```python
from build123d import *

# Parameters (mm, degrees)
AUFSATZ_LINEAR_AUSTRAGEN1_DEPTH      = 7.5
AUFSATZ_LINEAR_AUSTRAGEN1_DEPTH_BACK = 11
SKIZZE1_R                            = 12.5
SKIZZE1_R_2                          = 1.55
SCHNITT_LINEAR_AUSTRAGEN1_DEPTH      = 4.5
AUFSATZ_LINEAR_AUSTRAGEN2_DEPTH      = 5
SCHNITT_LINEAR_AUSTRAGEN4_DEPTH      = 22.650635095
SCHNITT_LINEAR_AUSTRAGEN4_DEPTH_BACK = 22.650635095
SCHNITT_LINEAR_AUSTRAGEN5_DEPTH      = 10
SCHNITT_LINEAR_AUSTRAGEN5_DEPTH_BACK = 22.650635095
SKIZZE5_OUTSIDE_W                    = 35.49
SKIZZE5_OUTSIDE_H                    = 35.49
SKIZZE5_OUTSIDE_W_2                  = 20
SKIZZE5_OUTSIDE_H_2                  = 30
VERRUNDUNG1_R                        = 1.2
VERRUNDUNG2_R                        = 1


with BuildPart() as part:
    # Skizze1 → Aufsatz-Linear austragen1 (new, two sides: drawn at the far end of the back side and taken through both)
    with BuildSketch(Plane.XY.offset(-AUFSATZ_LINEAR_AUSTRAGEN1_DEPTH_BACK)):
        Circle(SKIZZE1_R)
        with Locations((0, 8)):
            Circle(SKIZZE1_R_2, mode=Mode.SUBTRACT)
        with Locations(Location((0, -8, 0), (0, 0, 180))):
            Circle(SKIZZE1_R_2, mode=Mode.SUBTRACT)
    extrude(amount=AUFSATZ_LINEAR_AUSTRAGEN1_DEPTH + AUFSATZ_LINEAR_AUSTRAGEN1_DEPTH_BACK)

    # Skizze2 → Schnitt-Linear austragen1 (cut)
    with BuildSketch(Plane(origin=(0, 0, -11), x_dir=(-1, 0, 0), z_dir=(0, 0, -1))):
        with BuildLine():
            Line((-9, -4), (-9, 4))
            ThreePointArc((-9, 4), (-8.707106781, 4.707106781), (-8, 5))
            Line((-8, 5), (8, 5))
            ThreePointArc((8, 5), (8.707106781, 4.707106781), (9, 4))
            Line((9, 4), (9, -4))
            ThreePointArc((9, -4), (8.707106781, -4.707106781), (8, -5))
            Line((8, -5), (-8, -5))
            ThreePointArc((-8, -5), (-8.707106781, -4.707106781), (-9, -4))
        make_face()
    extrude(amount=-SCHNITT_LINEAR_AUSTRAGEN1_DEPTH, mode=Mode.SUBTRACT)

    # Skizze3 → Aufsatz-Linear austragen2 (add)
    with BuildSketch(Plane.XY.offset(7.5)):
        with BuildLine():
            Line((-8, 5), (8, 5))
            ThreePointArc((8, 5), (8.707106781, 4.707106781), (9, 4))
            Line((9, 4), (9, -4))
            ThreePointArc((9, -4), (8.707106781, -4.707106781), (8, -5))
            Line((8, -5), (-8, -5))
            ThreePointArc((-8, -5), (-8.707106781, -4.707106781), (-9, -4))
            Line((-9, -4), (-9, 4))
            ThreePointArc((-9, 4), (-8.707106781, 4.707106781), (-8, 5))
        make_face()
    extrude(amount=AUFSATZ_LINEAR_AUSTRAGEN2_DEPTH)

    # Skizze4 → Schnitt-Linear austragen4 (cut, two sides: drawn at the far end of the back side and taken through both)
    with BuildSketch(Plane.XY.offset(-SCHNITT_LINEAR_AUSTRAGEN4_DEPTH_BACK)):
        with BuildLine():
            Line((-6.5, -3), (6.5, -3))
            ThreePointArc((6.5, -3), (7.207106781, -2.707106781), (7.5, -2))
            Line((7.5, -2), (7.5, 2))
            ThreePointArc((7.5, 2), (7.207106781, 2.707106781), (6.5, 3))
            Line((6.5, 3), (-6.5, 3))
            ThreePointArc((-6.5, 3), (-7.207106781, 2.707106781), (-7.5, 2))
            Line((-7.5, 2), (-7.5, -2))
            ThreePointArc((-7.5, -2), (-7.207106781, -2.707106781), (-6.5, -3))
        make_face()
    extrude(amount=SCHNITT_LINEAR_AUSTRAGEN4_DEPTH + SCHNITT_LINEAR_AUSTRAGEN4_DEPTH_BACK, mode=Mode.SUBTRACT)

    # Skizze5 outside → Schnitt-Linear austragen5 (cut, two sides: drawn at the far end of the back side and taken through both)
    with BuildSketch(Plane.XY.offset(-SCHNITT_LINEAR_AUSTRAGEN5_DEPTH_BACK)):
        Rectangle(SKIZZE5_OUTSIDE_W, SKIZZE5_OUTSIDE_H)
        Rectangle(SKIZZE5_OUTSIDE_W_2, SKIZZE5_OUTSIDE_H_2, mode=Mode.SUBTRACT)
    extrude(amount=SCHNITT_LINEAR_AUSTRAGEN5_DEPTH + SCHNITT_LINEAR_AUSTRAGEN5_DEPTH_BACK, mode=Mode.SUBTRACT)

    # Verrundung1
    verrundung1_edges = [part.edges().sort_by_distance(p)[0] for p in [
        (-8.707106781, 4.707106781, -11),
        (-8.707106781, -4.707106781, -11),
        (0, -5, -11),
        (8.707106781, -4.707106781, -11),
        (8.707106781, 4.707106781, -11),
        (0, 5, -11),
    ]]
    fillet(verrundung1_edges, radius=VERRUNDUNG1_R)

    # Verrundung2
    verrundung2_edges = [part.edges().sort_by_distance(p)[0] for p in [
        (8.707106781, 4.707106781, 7.5),
        (0, 5, 7.5),
        (-8.707106781, 4.707106781, 7.5),
        (-9, 0, 7.5),
        (-8.707106781, -4.707106781, 7.5),
        (0, -5, 7.5),
        (8.707106781, -4.707106781, 7.5),
        (9, 0, 7.5),
    ]]
    fillet(verrundung2_edges, radius=VERRUNDUNG2_R - 0.0001)  # a hair under: the kernel refuses the full size


solid = part.part
```
The listing builds one solid part. Answer for the finished solid, in the listing's coordinates (mm). A direction names the side the tool comes from. Coordinates: 2 decimals unless noted, no trailing zeros. Write each loop counter-clockwise with the first axis right and the second up, starting at its lowest first coordinate (ties: lowest second). Pieces come first, ordered by that corner, then holes.
Q1. Section A-A, the plane x = 0 is taken. Write down the section's boundary in (y, z), then the cut area to 3 significant figures.
Returned:
outline: (-12.5, -11) - (-9.55, -11) - (-9.55, 7.5) - (-12.5, 7.5) - close; (-6.45, -11) - (-6.2, -11) arc R1.2 ccw to (-5, -9.8) - (-5, -6.5) - (-3, -6.5) - (-3, 12.5) - (-5, 12.5) - (-5, 8.5) arc R1 cw to (-6, 7.5) - (-6.45, 7.5) - close; (3, -6.5) - (5, -6.5) - (5, -9.8) arc R1.2 ccw to (6.2, -11) - (6.45, -11) - (6.45, 7.5) - (6, 7.5) arc R1 cw to (5, 8.5) - (5, 12.5) - (3, 12.5) - close; (9.55, -11) - (12.5, -11) - (12.5, 7.5) - (9.55, 7.5) - close
area: 239 mm2
Q2. Given P1, Ø1.2, axis at y = 0, z = 11, coming from the +X side; P2, Ø4, axis at x = -7.5, z = -2, coming from the -Y side (3 decimals); P3, Ø5, axis at x = -3.5, z = -8, coming from the -Y side, each flat-ended and moving along its own axis, determine where each tip first touches the part or whether it passes through.
Returned:
P1: stops at x = 9
P2: stops at y = -11.225
P3: stops at y = -12.46
Q3. Section D-D, the plane x = 6 is taken. Write down the section's boundary in (y, z).
Returned:
outline: (-10.97, -11) - (-6.2, -11) arc R1.2 ccw to (-5, -9.8) - (-5, -6.5) - (-3, -6.5) - (-3, 12.5) - (-5, 12.5) - (-5, 8.5) arc R1 cw to (-6, 7.5) - (-10.97, 7.5) - close; (3, -6.5) - (5, -6.5) - (5, -9.8) arc R1.2 ccw to (6.2, -11) - (10.97, -11) - (10.97, 7.5) - (6, 7.5) arc R1 cw to (5, 8.5) - (5, 12.5) - (3, 12.5) - close
Q4. Section C-C, the plane y = 8 is taken. Write down the section's boundary in (x, z), then the cut area to 3 significant figures.
Returned:
outline: (-9.6, -11) - (-1.55, -11) - (-1.55, 7.5) - (-9.6, 7.5) - close; (1.55, -11) - (9.6, -11) - (9.6, 7.5) - (1.55, 7.5) - close
area: 298 mm2
Q5. The mould has two halves that part along Y. Classify faces 1 (the cylindrical face through (-0.112, -5.301, 7.785)), 2 (the cylindrical face through (9.301, -0.056, 7.785)), 3 (the cylindrical face through (-0.112, 5.361, -10.658)): released by +Y, released by -Y, zero draft, split by the parting line, or undercut.
Returned:
face 1: released by -Y
face 2: zero draft
face 3: undercut
Q6. Which of the six approach directions +Z, -Z, +X, -X, +Y, -Y give full straight-line access (tool end or side, diameter ignored) to faces 4 (the flat face through (9, 0, 10)), 5 (the cylindrical face through (8.699, -4.715, -8.182)), 6 (the cylindrical face through (8.715, -4.699, 10.472)), 7 (the cylindrical face through (-7.215, -2.699, 2.867))?
Returned:
face 4: +Z, +X, +Y, -Y
face 5: -Z
face 6: +Z, +X, -Y
face 7: +Z, -Z
Q7. Section B-B, the plane z = 6.75 is taken. Write down the section's boundary in (x, y), then the cut area to 3 significant figures.
Returned:
outline: (-10, -7.5) arc R12.5 ccw to (10, -7.5) - (10, 7.5) arc R12.5 ccw to (-10, 7.5) - close; hole (-7.5, -2) arc R1 ccw to (-6.5, -3) - (6.5, -3) arc R1 ccw to (7.5, -2) - (7.5, 2) arc R1 ccw to (6.5, 3) - (-6.5, 3) arc R1 ccw to (-7.5, 2) - close; hole circle Ø3.1 at (0, -8); hole circle Ø3.1 at (0, 8)
area: 336 mm2
Q8. Find the intervals of material crossed by line 1 along X through (y, z) = (-0.5, -9); line 2 along Y through (x, z) = (2.75, 11.75); line 3 along X through (y, z) = (10, -5.75), in increasing order.
Returned:
line 1: x = -10 to -9, 9 to 10
line 2: y = -5 to -3, 3 to 5
line 3: x = -7.5 to 7.5
